Input: part model. Units: mm. Frame: model coordinates. A direction names the side the tool comes from. Coordinates: 2 decimals unless noted, no trailing zeros. Write each loop counter-clockwise with the first axis right and the second up, starting at its lowest first coordinate (ties: lowest second). Pieces come first, ordered by that corner, then holes. Notation, with made-up numbers: (87, 48.25) - (145, 48.25) arc R25 cw to (145, 76.25) - close; hole circle Ø7 at (78, 83.5). An arc over 180 degrees is marked (long way). Put each result on its own line as item: value. Start each with the question number.
1. Cut plane C-C, the plane z = 16.5. Return loops of the section in (x, y).
2. Line query: line 1 (Y direction, x = 153, z = 30.5); line 2 (X direction, y = 68.5, z = 77.5); line 3 (Y direction, x = 295, z = 66.5). Output: solid intervals per line, ascending.
3. Access query for faces 4 (the flat face through (143, 91, 30)), 5 (the flat face through (180, 0, 44)). Directions: +Z, -Z, +X, -X, +Y, -Y. A direction counts if a zero-diameter tool reaches every point of the face in a straight line with its end or side. Return the directions, or none.
4. Pull-direction query (Y, two-part tool) for faces 1 (the flat face through (0, 89, 44)), 2 (the flat face through (180, 180, 44)), 3 (the flat face through (25, 89, 60)); classes: released by +Y, released by -Y, zero draft, split by the parting line, or undercut.
5. Pin query (flat end, axial travel): pin 1 (2 mm diameter, centred on x = 69.5, y = 106.5, fed in from +Z). Return the tip coordinate at first contact, or that it passes through.
6. Cut plane A-A, the plane y = 90. Return loops of the section in (x, z), and give its area (4 significant figures).
7. Cut plane B-B, the plane x = 295. Return loops of the section in (y, z).
8. Cut plane D-D, the plane x = 84.5. Return loops of the section in (y, z), and give its area (3 significant figures).
from build123d import *

# Parameters (mm, degrees)
F0_W     = 365
F0_H     = 180
F1_DEPTH = 90
F2_W     = 240
F2_H     = 140
F3_DEPTH = 60
F4_R     = 20
F5_DEPTH = 90.001


with BuildPart() as f1:
    # F0 (on Top) → F1 (new body)
    with BuildSketch(Plane.XY):
        with Locations((182.5, 90)):
            Rectangle(F0_W, F0_H)
    extrude(amount=F1_DEPTH)

    # F2 (on face) → F3 (cut)
    with BuildSketch(Plane.XY.offset(90)):
        with Locations((145, 90)):
            Rectangle(F2_W, F2_H)
    extrude(amount=-F3_DEPTH, mode=Mode.SUBTRACT)

    # F4 (on face) → F5 (cut, through all)
    with BuildSketch(Plane.XY.offset(90)):
        with Locations((295, 90)):
            Circle(F4_R)
    extrude(amount=-F5_DEPTH, mode=Mode.SUBTRACT)


solid = f1.part
Report:
1. outline: (0, 0) - (365, 0) - (365, 180) - (0, 180) - close; hole circle Ø40 at (295, 90)
2. line 1: y = 0 to 20, 160 to 180
2. line 2: x = 0 to 25, 265 to 365
2. line 3: y = 0 to 70, 110 to 180
3. face 4: +Z
3. face 5: +Z, -Z, +X, -X, -Y
4. face 1: zero draft
4. face 2: released by +Y
4. face 3: undercut
5. pin 1: stops at z = 30
6. outline: (0, 0) - (275, 0) - (275, 90) - (265, 90) - (265, 30) - (25, 30) - (25, 90) - (0, 90) - close; (315, 0) - (365, 0) - (365, 90) - (315, 90) - close
6. area: 14,850 mm^2
7. outline: (0, 0) - (70, 0) - (70, 90) - (0, 90) - close; (110, 0) - (180, 0) - (180, 90) - (110, 90) - close
8. outline: (0, 0) - (180, 0) - (180, 90) - (160, 90) - (160, 30) - (20, 30) - (20, 90) - (0, 90) - close
8. area: 7,800 mm^2
